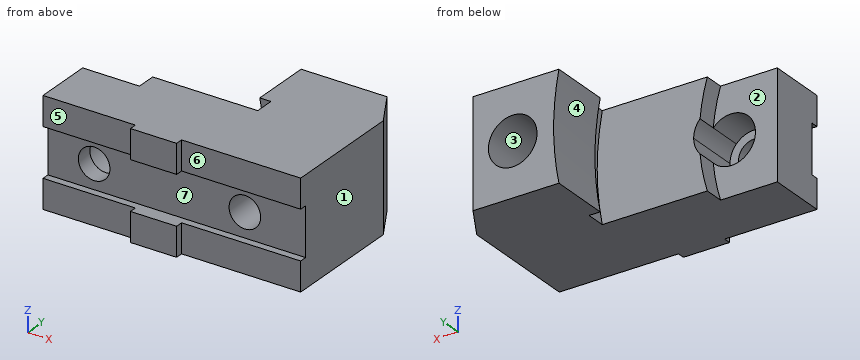
from build123d import *

# Parameters (mm, degrees)
BASE_DEPTH         = 44
MIDDLE_LEVEL_DEPTH = 8
UP_LEVEL_DEPTH     = 41
ANGLE_START        = 41
ANGLE_LEVEL_DEPTH  = 25
BIG_START          = 8
SKETCH2_7_R        = 6.5
BIG_CYL_DEPTH      = 22
SKETCH2_8_R        = 6.5
SMALL_CYL_DEPTH    = 28
SKETCH5_R          = 10
SKETCH5_R_2        = 6.5
BIG_CYL_2_DEPTH    = 22
SKETCH5_2_R        = 6.5
SMALL_CYL_2_DEPTH  = 69
BASE_ANGLE_DEPTH   = 45
SKETCH7_W          = 20
SKETCH7_H          = 6
DOWN_CUT_DEPTH     = 107


with BuildPart() as part:
    # Sketch1 → base (new body)
    with BuildSketch(Plane.XY):
        Polygon((-47.5, -12), (-47.5, 12), (58.5, 12), (58.5, -12), (9.5, -12), (9.5, -15), (-9.5, -15), (-9.5, -12), align=None)
    extrude(amount=-BASE_DEPTH)

    # Sketch2<4> → middle level (add)
    with BuildSketch(Plane(origin=(0, 12, 0), x_dir=(1, 0, 0), z_dir=(0, 1, 0))):
        with BuildLine():
            Line((14.5, 44), (-24.127153, 44))
            ThreePointArc((-24.127153, 44), (-22.234873, 36.459024), (-21.133434, 28.76267))
            ThreePointArc((-21.133434, 28.76267), (-19.181586, 25.628659), (-18.5, 22))
            ThreePointArc((-18.5, 22), (-19.181586, 18.371341), (-21.133434, 15.23733))
            ThreePointArc((-21.133434, 15.23733), (-22.234873, 7.540976), (-24.127153, 0))
            Line((-24.127153, 0), (14.5, 0))
            ThreePointArc((14.5, 0), (16.67208, 22), (14.5, 44))
        make_face()
        with BuildLine():
            Line((19.08509, 44), (14.5, 44))
            ThreePointArc((14.5, 44), (16.67208, 22), (14.5, 0))
            Line((14.5, 0), (19.08509, 0))
            ThreePointArc((19.08509, 0), (21.17208, 22), (19.08509, 44))
        make_face()
    extrude(amount=MIDDLE_LEVEL_DEPTH)

    # Sketch2 → up level (add)
    with BuildSketch(Plane(origin=(0, 12, 0), x_dir=(1, 0, 0), z_dir=(0, 1, 0))):
        with BuildLine():
            Line((58.5, 44), (19.08509, 44))
            ThreePointArc((19.08509, 44), (21.17208, 22), (19.08509, 0))
            Line((19.08509, 0), (58.5, 0))
            Line((58.5, 0), (58.5, 44))
        make_face()
    extrude(amount=UP_LEVEL_DEPTH)

    # Sketch2<6> → angle level (add)
    with BuildSketch(Plane(origin=(0, 12, 0), x_dir=(1, 0, 0), z_dir=(0, 1, 0)).offset(ANGLE_START)):
        with BuildLine():
            Line((19.08509, 44), (14.5, 44))
            ThreePointArc((14.5, 44), (16.67208, 22), (14.5, 0))
            Line((14.5, 0), (19.08509, 0))
            ThreePointArc((19.08509, 0), (21.17208, 22), (19.08509, 44))
        make_face()
    extrude(amount=-ANGLE_LEVEL_DEPTH)

    # Sketch2<7> → big cyl (cut)
    with BuildSketch(Plane(origin=(0, 12, 0), x_dir=(1, 0, 0), z_dir=(0, 1, 0)).offset(BIG_START)):
        with BuildLine():
            ThreePointArc((-18.5, 22), (-19.181586, 25.628659), (-21.133434, 28.76267))
            ThreePointArc((-21.133434, 28.76267), (-20.82792, 22), (-21.133434, 15.23733))
            ThreePointArc((-21.133434, 15.23733), (-19.181586, 18.371341), (-18.5, 22))
        make_face()
        with BuildLine():
            ThreePointArc((-21.133434, 15.23733), (-20.82792, 22), (-21.133434, 28.76267))
            ThreePointArc((-21.133434, 28.76267), (-38.5, 22), (-21.133434, 15.23733))
        make_face()
        with Locations((-28.5, 22)):
            Circle(SKETCH2_7_R, mode=Mode.SUBTRACT)
    extrude(amount=-BIG_CYL_DEPTH, mode=Mode.SUBTRACT)

    # Sketch2<8> → small cyl (cut, through all)
    with BuildSketch(Plane(origin=(0, 12, 0), x_dir=(1, 0, 0), z_dir=(0, 1, 0))):
        with Locations((-28.5, 22)):
            Circle(SKETCH2_8_R)
    extrude(amount=-SMALL_CYL_DEPTH, mode=Mode.SUBTRACT)

    # Sketch5 → big cyl 2 (cut)
    with BuildSketch(Plane(origin=(0, 53, 0), x_dir=(1, 0, 0), z_dir=(0, 1, 0))):
        with Locations((33.5, 22)):
            Circle(SKETCH5_R)
        with Locations((33.5, 22)):
            Circle(SKETCH5_R_2, mode=Mode.SUBTRACT)
    extrude(amount=-BIG_CYL_2_DEPTH, mode=Mode.SUBTRACT)

    # Sketch5<2> → small cyl 2 (cut, through all)
    with BuildSketch(Plane(origin=(0, 53, 0), x_dir=(1, 0, 0), z_dir=(0, 1, 0))):
        with Locations((33.5, 22)):
            Circle(SKETCH5_2_R)
    extrude(amount=-SMALL_CYL_2_DEPTH, mode=Mode.SUBTRACT)

    # Sketch6 → base angle (cut, through all)
    with BuildSketch(Plane.XY):
        Polygon((49.839746, 53), (58.5, 38), (58.5, 53), align=None)
    extrude(amount=-BASE_ANGLE_DEPTH, mode=Mode.SUBTRACT)

    # Sketch7 → down cut (cut, through all)
    with BuildSketch(Plane.ZY.offset(47.5)):
        with Locations((-22, -12)):
            Rectangle(SKETCH7_W, SKETCH7_H)
    extrude(amount=-DOWN_CUT_DEPTH, mode=Mode.SUBTRACT)


solid = part.part
CAD build for the part. Positions are in the model's coordinates, mm. Face numbers are marked on the shaded views. A direction names the side the tool comes from. Coordinates: 2 decimals unless noted, no trailing zeros. Loops run counter-clockwise (first coordinate to the right, second up) from the corner with the lowest first, then second, coordinate; pieces in that order, holes last. Notation, with made-up numbers: (-20.5, 24) -> (22.5, 24) arc R35 ccw to (22.5, 63) -> close; hole circle Ø10 at (40.5, 23.25). An arc over 180 degrees is marked (long way). One line per item, written item: value.
1. Slice it at B-B on y = 24. Write the cut outline in (x, z), and give its area (3 significant figures).
Answers:
outline: (19.09, -44) -> (58.5, -44) -> (58.5, 0) -> (19.09, 0) arc R117 cw to start; hole circle Ø13 at (33.5, -22)
area: 1,540 mm^2
2. Slice it at A-A on x = 33.5. Write the cut outline in (y, z).
Answers:
outline: (-12, -44) -> (53, -44) -> (53, -32) -> (31, -32) -> (31, -28.5) -> (-9, -28.5) -> (-9, -32) -> (-12, -32) -> close; (-12, -12) -> (-9, -12) -> (-9, -15.5) -> (31, -15.5) -> (31, -12) -> (53, -12) -> (53, 0) -> (-12, 0) -> close
3. Drill centre lines: line 1 (X direction, y = 16, z = -22); line 2 (Z direction, x = 33.5, y = 6); line 3 (Y direction, x = 19, z = -15.5). Where is each one in solid material? Low to high. Write a range as [from, to].
Answers:
line 1: x = [-18.5, 27], [40, 58.5]
line 2: z = [-44, -28.5], [-15.5, 0]
line 3: y = [-9, 20], [28, 53]
4. Flat gauge pins, fed straight in: P1, Ø8, axis at x = -3.5, z = -12, coming from the +Y side; P2, Ø3.5, axis at y = -14, z = -36, coming from the -X side; P3, Ø13, axis at x = -25.5, z = -38, coming from the -Y side; P4, Ø10.5, axis at x = -28.5, z = -22, coming from the +Y side. Where does each tip first touch, or does it go through?
Answers:
P1: stops at y = 20
P2: stops at x = -9.5
P3: stops at y = -12
P4: passes through
5. Slice it at C-C on x = 4.5. Write the cut outline in (y, z).
Answers:
outline: (-15, -44) -> (20, -44) -> (20, 0) -> (-15, 0) -> (-15, -12) -> (-9, -12) -> (-9, -32) -> (-15, -32) -> close
6. Slice it at D-D on y = -6.5. Write the cut outline in (x, z), and give its area (3 significant figures).
Answers:
outline: (-47.5, -44) -> (58.5, -44) -> (58.5, 0) -> (-47.5, 0) -> close; hole circle Ø13 at (-28.5, -22); hole circle Ø13 at (33.5, -22)
area: 4,400 mm^2
7. Which spindle directions (+Z, -Z, +X, -X, +Y, -Y) get a long thin tool onto all of the face, cutting with end or side? Do the marked faces 5, 6 and 7. Say none if no direction does.
Answers:
face 5: +Z, -Z, -X, -Y
face 6: +Z, -Z, +X, -Y
face 7: +X, -X, -Y
8. Pull direction X, two halves, no side cores. Call the marked faces 1, 2, 3 and 4: pulls with the +X half, pulls with the -X half, needs draft (parallel to the pull), parting line crosses it, or undercut.
Answers:
face 1: pulls with the +X half
face 2: needs draft
face 3: undercut
face 4: pulls with the -X half
